For this review, use the dimensioned drawing (mm, ordinates from the lowest corner) and the shaded views. A direction names the side the tool comes from. Coordinates: 2 decimals unless noted, no trailing zeros. Loops run counter-clockwise (first coordinate to the right, second up) from the corner with the lowest first, then second, coordinate; pieces in that order, holes last. Notation, with made-up numbers: M 34,5 L 92,5 A22 ccw 92,17 Z; hole C -19.5,62.25 d8. An arc over 180 degrees is marked long. One line per item, written item: value.
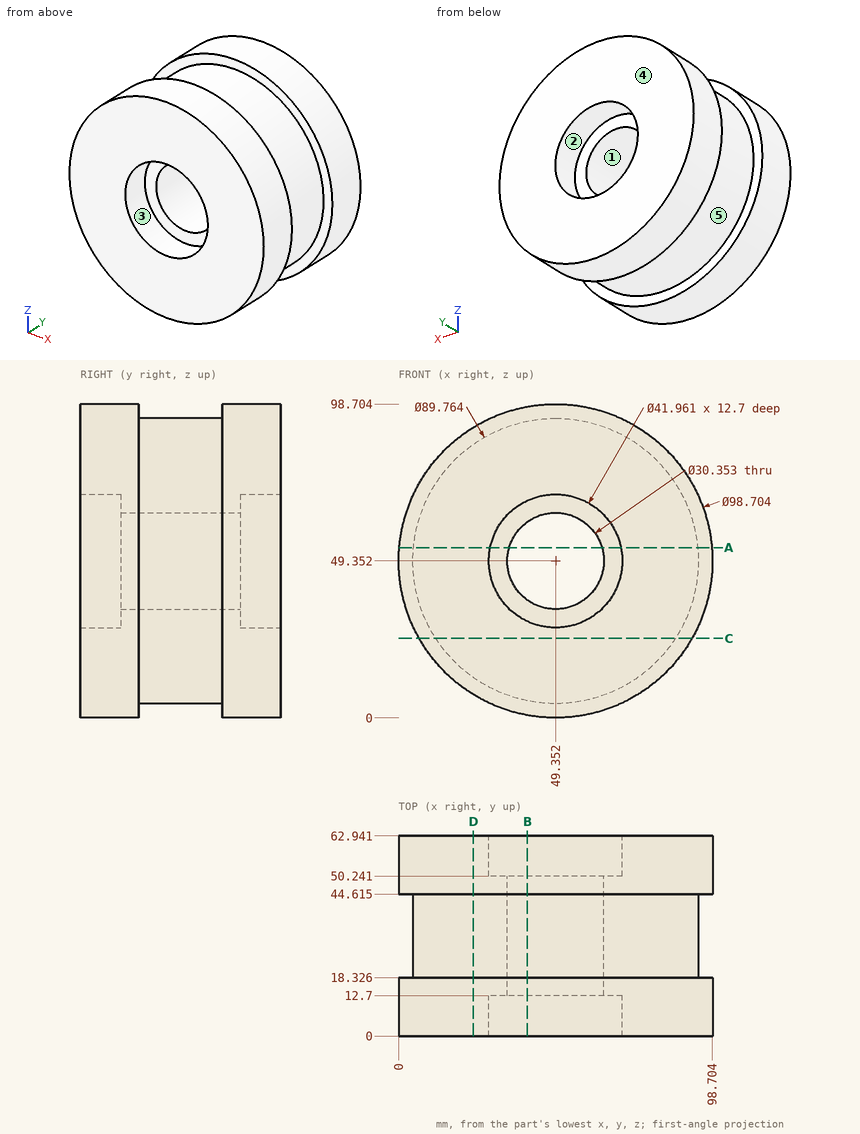
(1) Draft analysis for pull direction Z (two halves, no side actions). For the marked faces 3, 4 and 5, state which applies: pulls with the +Z half, pulls with the -Z half, needs draft (parallel to the pull), parting line crosses it, or undercut.
Checks:
face 3: undercut
face 4: needs draft
face 5: parting line crosses it
(2) Add section C-C on z = 25. State the section outline as (x, y) points (1 decimal).
Checks:
outline: M 6.4,0 L 92.3,0 L 92.3,18.3 L 87.1,18.3 L 87.1,44.6 L 92.3,44.6 L 92.3,62.9 L 6.4,62.9 L 6.4,44.6 L 11.7,44.6 L 11.7,18.3 L 6.4,18.3 Z
(3) Add section A-A on z = 53.5. State the section outline as (x, y) points (1 decimal).
Checks:
outline: M 0.2,0 L 28.8,0 L 28.8,12.7 L 34.8,12.7 L 34.8,50.2 L 28.8,50.2 L 28.8,62.9 L 0.2,62.9 L 0.2,44.6 L 4.7,44.6 L 4.7,18.3 L 0.2,18.3 Z; M 64,12.7 L 69.9,12.7 L 69.9,0 L 98.5,0 L 98.5,18.3 L 94,18.3 L 94,44.6 L 98.5,44.6 L 98.5,62.9 L 69.9,62.9 L 69.9,50.2 L 64,50.2 Z
(4) Add section B-B on x = 40.5. State the section outline as (y, z) points (1 decimal).
Checks:
outline: M 0,0.8 L 18.3,0.8 L 18.3,5.4 L 44.6,5.4 L 44.6,0.8 L 62.9,0.8 L 62.9,30.3 L 50.2,30.3 L 50.2,37 L 12.7,37 L 12.7,30.3 L 0,30.3 Z; M 0,68.4 L 12.7,68.4 L 12.7,61.7 L 50.2,61.7 L 50.2,68.4 L 62.9,68.4 L 62.9,97.9 L 44.6,97.9 L 44.6,93.4 L 18.3,93.4 L 18.3,97.9 L 0,97.9 Z
(5) Tool access review of the marked faces 1 and 2: name each direction out of +Z, -Z, +X, -X, +Y, -Y from which nothing blocks a thin tool from reaching the whole face with its end or side.
Checks:
face 1: +Y, -Y
face 2: +Y
(6) Add section D-D on x = 23.5. State the section outline as (y, z) points (1 decimal), then the cut area to 3 significant figures.
Checks:
outline: M 0,7.3 L 18.3,7.3 L 18.3,12.7 L 44.6,12.7 L 44.6,7.3 L 62.9,7.3 L 62.9,91.4 L 44.6,91.4 L 44.6,86 L 18.3,86 L 18.3,91.4 L 0,91.4 Z
area: 5,010 mm^2
(7) To check wall thickness, follow L1, parallel to Y at x = 24, z = 9 (1 decimal); L2, parallel to Y at x = 31.5, z = 58.5; L3, parallel to X at y = 21.5, z = 54.5 (1 decimal). State the ranges of each line that lie inside material, in increasing order. Write a range as [from, to].
Checks:
L1: [0, 18.3], [44.6, 62.9]
L2: [12.7, 50.24]
L3: [4.8, 35.1], [63.6, 93.9]
(8) Insertion check: pin 1 Ø2 at (x, y) = (40.5, 55.5) entering from +Z; pin 2 Ø1.5 at (x, y) = (71.5, 45.5) entering from -Z; pin 3 Ø2 at (y, z) = (27, 35.5) entering from +X (1 decimal); pin 4 Ø6 at (x, z) = (67, 44) entering from -Y. Each pin has a flat end and moves straight along its axis. Give the tip position at first contact, or say it passes through.
Checks:
pin 1: z = 98.08
pin 2: z = 4.88
pin 3: x = 92.4
pin 4: y = 0
